Verification items for the finished model (mm, model axes). A direction names the side the tool comes from. Coordinates: 2 decimals unless noted, no trailing zeros. Order: outer loops, then holes, each group sorted by start corner. A loop starts at its lowest first (then second) coordinate and runs counter-clockwise, first axis right, second up. Notation, with made-up numbers: M 71.5,-6 L 82.5,-6 A3 ccw 82.5,-2 Z; hole C 0.25,76 d6. An arc over 180 degrees is marked long. Return JSON: item names as keys, results as strings. Group by question number.
1. Section check D-D, the plane z = 19. Record the cut outline in (x, y).
2. Section check C-C, the plane y = 20. Give the number of separate pieces and of enclosed holes in the cut face, plus the area to 3 significant figures.
3. Material ranges on line 1 along X through (y, z) = (4.75, -15); line 2 along X through (y, z) = (14.25, -2.5); line 3 along Z through (x, y) = (0, 8.75), recorded low to high.
4. Mould release check, pull along Y, two halves, no side actions. Record for faces 6 (the flat face through (-5, 5, -16)), 7 (the cylindrical face through (16.97, 10.57, -8.1)), 8 (the flat face through (0, 5, -20)): +Y half, -Y half, draft (parallel to the pull), parting line (faces both ways), or undercut.
5. Section check A-A, the plane x = 0. Record the cut outline in (y, z), plus the area to 3 significant figures.
6. Gauge pin test, flat ends, axial feed: pin 1 (3 mm diameter, centred on y = 5, z = -5, fed in from +X); pin 2 (4 mm diameter, centred on y = 14, z = 1, fed in from -X); pin 3 (1.5 mm diameter, centred on x = -5.5, y = 4, fed in from -Z). Record the tip position at first contact, or that the pin passes through.
7. Section check B-B, the plane y = 4. Record the cut outline in (x, z).
8. Set-up check for faces 1 (the cylindrical face through (0.66, 8.521, -14.985)), 2 (the cylindrical face through (2.615, 5.751, -18.028)), 3 (the cylindrical face through (17.48, 22.93, -0.65)), 4 (the flat face through (-17, 17, -7.5)), 5 (the cylindrical face through (-18.028, 5.751, -2.615)): record each of +Z, -Z, +X, -X, +Y, -Y from which the full face is reachable in a straight line by a thin tool's end or side.
```python
from build123d import *

# Parameters (mm, degrees)
SKETCH1_R                = 22
BOSS_EXTRUDE1_DEPTH      = 10
SKETCH5_R                = 15
CUT_EXTRUDE3_DEPTH       = 5
CUT_EXTRUDE5_START       = -3
SKETCH7_R                = 15
CUT_EXTRUDE5_DEPTH       = 3
SKETCH8_R                = 7.5
CUT_EXTRUDE6_DEPTH       = 3
SKETCH6_R                = 2.5
CUT_EXTRUDE7_DEPTH       = 10
SKETCH9_W                = 6.833639819
SKETCH9_H                = 40.698121589
SKETCH9_W_2              = 26.089318242
SKETCH9_H_2              = 6.104718238
CUT_EXTRUDE8_DEPTH       = 10
BOSS_EXTRUDE3_DEPTH      = 15
FILLET1_R                = 2
FILLET2_R                = 10
CUT_EXTRUDE9_DEPTH       = 42
CUT_EXTRUDE9_DEPTH_BACK  = 15
SKETCH11_R               = 3
FILLET3_START            = 9
FILLET3_DEPTH            = 16
FILLET3_START_2          = -21
FILLET3_2_DEPTH          = 42
FILLET4_R                = 2
CUT_EXTRUDE18_DEPTH      = 30.2
CUT_EXTRUDE18_DEPTH_BACK = 0.2
FILLET5_R                = 20
SKETCH14_R               = 3
SKETCH14_R_2             = 2.5
BOSS_EXTRUDE4_DEPTH      = 0.8
BOSS_EXTRUDE5_START      = -0.8
SKETCH15_R               = 3
SKETCH15_R_2             = 2.5
BOSS_EXTRUDE5_DEPTH      = 0.8
SKETCH17_R               = 2.5
CUT_EXTRUDE20_DEPTH      = 4
SKETCH18_R               = 2.5
CUT_EXTRUDE21_DEPTH      = 4


with BuildPart() as part:
    # Sketch1 → Boss-Extrude1 (new body)
    with BuildSketch(Plane(origin=(0, 0, 0), x_dir=(1, 0, 0), z_dir=(0, 1, 0))):
        with Locations(Location((0, 0, 0), (0, 0, 270))):
            Circle(SKETCH1_R)
    extrude(amount=BOSS_EXTRUDE1_DEPTH)

    # Sketch5 → Cut-Extrude3 (cut)
    with BuildSketch(Plane(origin=(0, 10, 0), x_dir=(1, 0, 0), z_dir=(0, 1, 0))):
        with Locations(Location((0, 0, 0), (0, 0, 270))):
            Circle(SKETCH5_R)
    extrude(amount=-CUT_EXTRUDE3_DEPTH, mode=Mode.SUBTRACT)

    # Sketch7 → Cut-Extrude5 (cut)
    with BuildSketch(Plane(origin=(0, 0, 0), x_dir=(-1, 0, 0), z_dir=(0, -1, 0)).offset(CUT_EXTRUDE5_START)):
        with Locations(Location((0, 0, 0), (0, 0, 270))):
            Circle(SKETCH7_R)
    extrude(amount=CUT_EXTRUDE5_DEPTH, mode=Mode.SUBTRACT)

    # Sketch8 → Cut-Extrude6 (cut)
    with BuildSketch(Plane(origin=(0, 3, 0), x_dir=(-1, 0, 0), z_dir=(0, -1, 0))):
        with Locations(Location((0, 0, 0), (0, 0, 90))):
            Circle(SKETCH8_R)
    extrude(amount=-CUT_EXTRUDE6_DEPTH, mode=Mode.SUBTRACT)

    # Sketch6 → Cut-Extrude7 (cut)
    with BuildSketch(Plane(origin=(0, 10, 0), x_dir=(1, 0, 0), z_dir=(0, 1, 0))):
        with Locations(Location((13.081475452, 13.081475452, 0), (0, 0, 270))):
            Circle(SKETCH6_R)
        with Locations(Location((-13.081475452, -13.081475452, 0), (0, 0, 270))):
            Circle(SKETCH6_R)
        with Locations(Location((-13.081475452, 13.081475452, 0), (0, 0, 270))):
            Circle(SKETCH6_R)
        with Locations(Location((13.081475452, -13.081475452, 0), (0, 0, 270))):
            Circle(SKETCH6_R)
    extrude(amount=-CUT_EXTRUDE7_DEPTH, mode=Mode.SUBTRACT)

    # Sketch9 → Cut-Extrude8 (cut)
    with BuildSketch(Plane(origin=(0, 10, 0), x_dir=(1, 0, 0), z_dir=(0, 1, 0))):
        with Locations((-23.416819909, -5.65916064)):
            Rectangle(SKETCH9_W, SKETCH9_H)
        with Locations((-0.506301064, 23.052359119)):
            Rectangle(SKETCH9_W_2, SKETCH9_H_2)
    extrude(amount=-CUT_EXTRUDE8_DEPTH, mode=Mode.SUBTRACT)

    # Sketch10 → Boss-Extrude3 (add)
    with BuildSketch(Plane(origin=(0, 10, 0), x_dir=(1, 0, 0), z_dir=(0, 1, 0))):
        Polygon((-15, -7.5), (-15, 7.5), (-19, 7.5), (-19, 5.5), (-20, 5.5), (-20, 3.5), (-19, 3.5), (-19, -3.5), (-20, -3.5), (-20, -5.5), (-19, -5.5), (-19, -7.5), align=None)
        Polygon((20, -5.5), (20, -3.5), (19, -3.5), (19, 3.5), (20, 3.5), (20, 5.5), (19, 5.5), (19, 7.5), (15, 7.5), (15, -7.5), (19, -7.5), (19, -5.5), align=None)
    extrude(amount=BOSS_EXTRUDE3_DEPTH)

    # Fillet1
    fillet1_edges = [part.edges().sort_by_distance(p)[0] for p in [
        (-17, 10, -7.5),
        (-17, 25, -7.5),
        (-17, 10, 7.5),
        (-17, 25, 7.5),
        (17, 10, -7.5),
        (17, 10, 7.5),
        (17, 25, -7.5),
        (17, 25, 7.5),
    ]]
    fillet(fillet1_edges, radius=FILLET1_R)

    # Fillet2
    # the kernel refuses this fillet: 10 mm, written as the material it adds along each edge
    with BuildSketch(Plane(origin=(-19, 10, -14.397247359), x_dir=(0, 1, 0), z_dir=(0, 0, 1))) as fillet2_piece_1_section:
        with BuildLine():
            CenterArc((4.358898944, 10), FILLET2_R, 244.158067237, 25.841932763)
            Line((0, 1), (0, 0))
            Line((0, 0), (4.358898944, 0))
        make_face()
    fillet2_piece_1 = extrude(amount=28.794494718, mode=Mode.PRIVATE)
    fillet2_piece_1 = split(fillet2_piece_1, bisect_by=Plane(origin=(-19, 10, -5.5), z_dir=(0, 0, 1)), keep=Keep.TOP, mode=Mode.PRIVATE)
    fillet2_piece_1 = split(fillet2_piece_1, bisect_by=Plane(origin=(-19, 10, 5.5), z_dir=(0, 0, -1)), keep=Keep.TOP, mode=Mode.PRIVATE)
    add(fillet2_piece_1)

    # Sketch11 → Cut-Extrude9 (cut, two sides: drawn at the far end of the back side and taken through both)
    with BuildSketch(Plane(origin=(-15, 0, 0), x_dir=(0, 0, -1), z_dir=(1, 0, 0)).offset(-CUT_EXTRUDE9_DEPTH_BACK)):
        with Locations(Location((0, 20, 0), (0, 0, 180))):
            Circle(SKETCH11_R)
    extrude(amount=CUT_EXTRUDE9_DEPTH + CUT_EXTRUDE9_DEPTH_BACK, mode=Mode.SUBTRACT)

    # Fillet3: read off the stored shape, not the designer's step
    # Fillet3 outline → Fillet3 (add)
    with BuildSketch(Plane(origin=(0, 0, 0), x_dir=(1, 0, 0), z_dir=(0, 1, 0)).offset(FILLET3_START)):
        with BuildLine():
            Line((19, -5.5), (19, -7.232050808))
            ThreePointArc((19, -7.232050808), (19.267949192, -6.232050808), (20, -5.5))
            Line((20, -5.5), (19, -5.5))
        make_face()
        with BuildLine():
            Line((19, 5.5), (20, 5.5))
            ThreePointArc((20, 5.5), (19.267949192, 6.232050808), (19, 7.232050808))
            Line((19, 7.232050808), (19, 5.5))
        make_face()
        with BuildLine():
            ThreePointArc((-19, 7.232050808), (-19.267949192, 6.232050808), (-20, 5.5))
            Line((-20, 5.5), (-19, 5.5))
            Line((-19, 5.5), (-19, 7.232050808))
        make_face()
        with BuildLine():
            ThreePointArc((-20, -5.5), (-19.267949192, -6.232050808), (-19, -7.232050808))
            Line((-19, -7.232050808), (-19, -5.5))
            Line((-19, -5.5), (-20, -5.5))
        make_face()
    extrude(amount=FILLET3_DEPTH)

    # Fillet3 2 outline → Fillet3 2 (cut)
    with BuildSketch(Plane.YZ.offset(FILLET3_START_2)):
        with BuildLine():
            ThreePointArc((25, -5.5), (24.732050807, -6.5), (23.999999999, -7.232050808))
            Line((23.999999999, -7.232050808), (25, -7.232050808))
            Line((25, -7.232050808), (25, -5.5))
        make_face()
        with BuildLine():
            ThreePointArc((23.999999999, 7.232050808), (24.732050807, 6.5), (25, 5.5))
            Line((25, 5.5), (25, 7.232050808))
            Line((25, 7.232050808), (23.999999999, 7.232050808))
        make_face()
    extrude(amount=FILLET3_2_DEPTH, mode=Mode.SUBTRACT)

    # Fillet4
    fillet4_edges = [part.edges().sort_by_distance(p)[0] for p in [
        (0, 3, -15),
        (0, 5, -15),
    ]]
    fillet(fillet4_edges, radius=FILLET4_R)

    # Sketch13 → Cut-Extrude18 (cut, two sides: drawn at the far end of the back side and taken through both)
    with BuildSketch(Plane.ZY.offset(-15).offset(-CUT_EXTRUDE18_DEPTH_BACK)):
        with BuildLine():
            ThreePointArc((-1.041889066, 14.091153482), (-4.242640687, 15.757359313), (-5.908846518, 18.958110934))
            ThreePointArc((-5.908846518, 18.958110934), (-5.513931092, 22.365705796), (-3.31662479, 25))
            Line((-3.31662479, 25), (-5.5, 25))
            ThreePointArc((-5.5, 25), (-6.914213562, 24.414213562), (-7.5, 23))
            Line((-7.5, 23), (-7.5, 12.759289849))
            ThreePointArc((-7.5, 12.759289849), (-6.78111068, 12.755479981), (-6.066925886, 12.837677605))
            Line((-6.066925886, 12.837677605), (0, 13.907440329))
            Line((0, 13.907440329), (-1.041889066, 14.091153482))
        make_face()
        with BuildLine():
            ThreePointArc((2.954423259, 19.479055467), (0, 17), (-2.954423259, 19.479055467))
            Line((-2.954423259, 19.479055467), (-5.908846518, 18.958110934))
            ThreePointArc((-5.908846518, 18.958110934), (-4.242640687, 15.757359313), (-1.041889066, 14.091153482))
            Line((-1.041889066, 14.091153482), (0, 13.907440329))
            Line((0, 13.907440329), (1.041889066, 14.091153482))
            ThreePointArc((1.041889066, 14.091153482), (4.242640687, 15.757359313), (5.908846518, 18.958110934))
            Line((5.908846518, 18.958110934), (2.954423259, 19.479055467))
        make_face()
        with BuildLine():
            Line((-5.908846518, 18.958110934), (-2.954423259, 19.479055467))
            ThreePointArc((-2.954423259, 19.479055467), (-0.261467228, 22.988584094), (3, 20))
            ThreePointArc((3, 20), (2.988584094, 19.738532772), (2.954423259, 19.479055467))
            Line((2.954423259, 19.479055467), (5.908846518, 18.958110934))
            ThreePointArc((5.908846518, 18.958110934), (5.513931092, 22.365705796), (3.31662479, 25))
            Line((3.31662479, 25), (-3.31662479, 25))
            ThreePointArc((-3.31662479, 25), (-5.513931092, 22.365705796), (-5.908846518, 18.958110934))
        make_face()
        with BuildLine():
            Line((-2.954423259, 19.479055467), (0, 20))
            Line((0, 20), (2.954423259, 19.479055467))
            ThreePointArc((2.954423259, 19.479055467), (2.988584094, 19.738532772), (3, 20))
            ThreePointArc((3, 20), (-0.261467228, 22.988584094), (-2.954423259, 19.479055467))
        make_face()
        with BuildLine():
            Line((2.954423259, 19.479055467), (0, 20))
            Line((0, 20), (-2.954423259, 19.479055467))
            ThreePointArc((-2.954423259, 19.479055467), (0, 17), (2.954423259, 19.479055467))
        make_face()
        with BuildLine():
            ThreePointArc((3.31662479, 25), (5.513931092, 22.365705796), (5.908846518, 18.958110934))
            ThreePointArc((5.908846518, 18.958110934), (4.242640687, 15.757359313), (1.041889066, 14.091153482))
            Line((1.041889066, 14.091153482), (0, 13.907440329))
            Line((0, 13.907440329), (5.162816476, 12.997096488))
            ThreePointArc((5.162816476, 12.997096488), (6.333883164, 12.907333738), (7.5, 13.047426789))
            Line((7.5, 13.047426789), (7.5, 23))
            ThreePointArc((7.5, 23), (6.914213562, 24.414213562), (5.5, 25))
            Line((5.5, 25), (3.31662479, 25))
        make_face()
    extrude(amount=CUT_EXTRUDE18_DEPTH + CUT_EXTRUDE18_DEPTH_BACK, mode=Mode.SUBTRACT)

    # Fillet5
    fillet5_edges = [part.edges().sort_by_distance(p)[0] for p in [
        (15.1, 13.907440329, 0),
        (-15.1, 13.907440329, 0),
    ]]
    fillet(fillet5_edges, radius=FILLET5_R)

    # Sketch14 → Boss-Extrude4 (add)
    with BuildSketch(Plane.ZY.offset(-15.2)):
        with Locations((0, 20)):
            Circle(SKETCH14_R)
        with Locations((0, 20)):
            Circle(SKETCH14_R_2, mode=Mode.SUBTRACT)
    extrude(amount=-BOSS_EXTRUDE4_DEPTH)

    # Sketch15 → Boss-Extrude5 (add)
    with BuildSketch(Plane(origin=(-15.2, 0, 0), x_dir=(0, 0, -1), z_dir=(1, 0, 0)).offset(BOSS_EXTRUDE5_START)):
        with Locations(Location((0, 20, 0), (0, 0, 180))):
            Circle(SKETCH15_R)
        with Locations(Location((0, 20, 0), (0, 0, 180))):
            Circle(SKETCH15_R_2, mode=Mode.SUBTRACT)
    extrude(amount=BOSS_EXTRUDE5_DEPTH)

    # Sketch17 → Cut-Extrude20 (cut)
    with BuildSketch(Plane(origin=(0, 0, -20), x_dir=(-1, 0, 0), z_dir=(0, 0, -1))):
        with Locations((-5, 5)):
            Circle(SKETCH17_R)
        with Locations((5, 5)):
            Circle(SKETCH17_R)
    extrude(amount=-CUT_EXTRUDE20_DEPTH, mode=Mode.SUBTRACT)

    # Sketch18 → Cut-Extrude21 (cut)
    with BuildSketch(Plane.ZY.offset(20)):
        with Locations((-5, 5)):
            Circle(SKETCH18_R)
        with Locations((5, 5)):
            Circle(SKETCH18_R)
    extrude(amount=-CUT_EXTRUDE21_DEPTH, mode=Mode.SUBTRACT)


solid = part.part
```
Answers follow:
{
 "1": {"outline": "M -11.09,0 L 11.09,0 L 11.09,10 L -11.09,10 Z"},
 "2": {"separate pieces": "4", "enclosed holes": "0", "area": "80.0 mm^2"},
 "3": {"line 1": "-16.09 to -14.68, -11.48 to 11.48, 14.68 to 16.09", "line 2": "-19 to -15.2, 15.2 to 19", "line 3": "-20 to -15, 15 to 22"},
 "4": {"face 6": "undercut", "face 7": "+Y half", "face 8": "draft"},
 "5": {"outline": "M 0,-20 L 10,-20 L 10,-15 L 7,-15 A2 cw 5,-13 L 5,-7.5 L 3,-7.5 L 3,-13 A2 cw 1,-15 L 0,-15 Z; M 0,15 L 1,15 A2 cw 3,13 L 3,7.5 L 5,7.5 L 5,13 A2 cw 7,15 L 10,15 L 10,22 L 0,22 Z", "area": "153 mm^2"},
 "6": {"pin 1": "x = 21.72", "pin 2": "x = -19.28", "pin 3": "z = -16"},
 "7": {"outline": "M -20,-9.17 A22 ccw -9.17,-20 L -7.29,-20 L -7.29,-16 L -2.71,-16 L -2.71,-20 L 2.71,-20 L 2.71,-16 L 7.29,-16 L 7.29,-20 L 9.17,-20 A22 ccw long -20,9.17 L -20,7.29 L -16,7.29 L -16,2.71 L -20,2.71 L -20,-2.71 L -16,-2.71 L -16,-7.29 L -20,-7.29 Z; hole C -13.08,-13.08 d5; hole C -13.08,13.08 d5; hole C 0,0 d15; hole C 13.08,-13.08 d5; hole C 13.08,13.08 d5"},
 "8": {"face 1": "+Y", "face 2": "-Z", "face 3": "+X", "face 4": "-Z, +X, -X, +Y", "face 5": "-X"}
}
